```python
from build123d import *
from OCP.BRepFilletAPI import BRepFilletAPI_MakeChamfer

# Parameters (mm, degrees)
SKETCH1_W           = 22
SKETCH1_H           = 72
BOSS_EXTRUDE1_DEPTH = 5
SKETCH2_W           = 7
SKETCH2_H           = 15
BOSS_EXTRUDE2_DEPTH = 40
CHAMFER1_SIZE       = 1
FILLET1_R           = 10
CUT_EXTRUDE2_DEPTH  = 59.668560575
SKETCH6_W           = 7.5
SKETCH6_H           = 7.5
CUT_EXTRUDE3_DEPTH  = 55.927224579
CHAMFER2_SIZE2      = 15
CHAMFER2_SIZE       = 7.5
CHAMFER7_SIZE       = 7.5
CHAMFER3_SIZE       = 5
CUT_EXTRUDE6_DEPTH  = 2
CUT_EXTRUDE7_DEPTH  = 4
CHAMFER4_SIZE       = 2
CHAMFER4_SIZE_2     = 0.727940469
CUT_EXTRUDE8_DEPTH  = 60.42432162
CHAMFER8_SIZE2      = 7.5
CHAMFER8_SIZE       = 15
SKETCH12_R          = 1.7145
CUT_EXTRUDE9_DEPTH  = 60.42432162
SKETCH13_R          = 1.7145
CUT_EXTRUDE10_DEPTH = 55.927224579


with BuildPart() as part:
    # Sketch1 → Boss-Extrude1 (new body)
    with BuildSketch(Plane(origin=(0, 0, 0), x_dir=(1, 0, 0), z_dir=(0, 1, 0))):
        Rectangle(SKETCH1_W, SKETCH1_H)
    extrude(amount=BOSS_EXTRUDE1_DEPTH)

    # Sketch2 → Boss-Extrude2 (add)
    with BuildSketch(Plane(origin=(0, 5, 0), x_dir=(1, 0, 0), z_dir=(0, 1, 0))):
        with Locations((0, -28.5)):
            Rectangle(SKETCH2_W, SKETCH2_H)
    extrude(amount=BOSS_EXTRUDE2_DEPTH)

    # Chamfer1
    chamfer1_edges = [part.edges().sort_by_distance(p)[0] for p in [
        (0, 45, 36),
        (0, 45, 21),
    ]]
    chamfer(chamfer1_edges, length=CHAMFER1_SIZE)

    # Fillet1
    fillet1_edges = [part.edges().sort_by_distance(p)[0] for p in [
        (0, 5, 21),
    ]]
    fillet(fillet1_edges, radius=FILLET1_R)

    # Sketch5 → Cut-Extrude2 (cut, through all)
    with BuildSketch(Plane.XZ):
        with BuildLine():
            Line((3.4, 2), (3.4, -18))
            ThreePointArc((3.4, -18), (0, -21.4), (-3.4, -18))
            Line((-3.4, -18), (-3.4, 2))
            ThreePointArc((-3.4, 2), (0, 5.4), (3.4, 2))
        make_face()
    extrude(amount=-CUT_EXTRUDE2_DEPTH, mode=Mode.SUBTRACT)

    # Sketch6 → Cut-Extrude3 (cut, through all)
    with BuildSketch(Plane(origin=(0, 5, 0), x_dir=(1, 0, 0), z_dir=(0, 1, 0))):
        with Locations((7.25, -32.25)):
            Rectangle(SKETCH6_W, SKETCH6_H)
    cut_extrude3 = extrude(amount=-CUT_EXTRUDE3_DEPTH, mode=Mode.SUBTRACT)

    # Mirror1: Cut-Extrude3 across plane
    add(cut_extrude3.mirror(Plane(origin=(0, 0, 0), x_dir=(0, 0, 1), z_dir=(1, 0, 0))), mode=Mode.SUBTRACT)

    # Chamfer2
    chamfer2_edges = [part.edges().sort_by_distance(p)[0] for p in [
        (11, 2.5, 28.5),
    ]]
    chamfer2_side = [part.faces().sort_by_distance(p)[0] for p in [
        (10.85, 2.5, 28.5),
    ]]
    chamfer(chamfer2_edges, length=CHAMFER2_SIZE - 0.0001, length2=CHAMFER2_SIZE2 - 0.0001, reference=chamfer2_side[0])  # a hair under: the kernel refuses the full size

    # Chamfer7
    chamfer7_edges = [part.edges().sort_by_distance(p)[0] for p in [
        (0, 0, 36),
    ]]
    chamfer(chamfer7_edges, length=CHAMFER7_SIZE)

    # Chamfer3
    chamfer3_edges = [part.edges().sort_by_distance(p)[0] for p in [
        (-11, 2.5, -36),
        (11, 2.5, -36),
    ]]
    chamfer(chamfer3_edges, length=CHAMFER3_SIZE)

    # Sketch8 → Cut-Extrude6 (cut)
    # profile 1 of 2: a face of its own
    with BuildSketch(Plane.XZ):
        with BuildLine():
            Line((8.5, -18), (8.5, 2))
            ThreePointArc((8.5, 2), (0.500870333, 10.485230045), (-8.440971508, 3))
            Line((-8.440971508, 3), (-6, 3))
            Line((-6, 3), (-6, -19))
            Line((-6, -19), (-8.440971508, -19))
            ThreePointArc((-8.440971508, -19), (0.500870333, -26.485230045), (8.5, -18))
        make_face()
        with BuildLine():
            Line((-3.4, -18), (-3.4, 2))
            ThreePointArc((-3.4, 2), (0, 5.4), (3.4, 2))
            Line((3.4, 2), (3.4, -18))
            ThreePointArc((3.4, -18), (0, -21.4), (-3.4, -18))
        make_face(mode=Mode.SUBTRACT)
    # profile 2 of 2: a face of its own
    with BuildSketch(Plane.XZ):
        with BuildLine():
            Line((-6, 3), (-8.440971508, 3))
            ThreePointArc((-8.440971508, 3), (-8.485230045, 2.500870333), (-8.5, 2))
            Line((-8.5, 2), (-8.5, -18))
            ThreePointArc((-8.5, -18), (-8.485230045, -18.500870333), (-8.440971508, -19))
            Line((-8.440971508, -19), (-6, -19))
            Line((-6, -19), (-6, 3))
        make_face()
    extrude(amount=-CUT_EXTRUDE6_DEPTH, mode=Mode.SUBTRACT)

    # Sketch8<3> → Cut-Extrude7 (cut)
    with BuildSketch(Plane.XZ):
        with BuildLine():
            Line((-6, 3), (-8.440971508, 3))
            ThreePointArc((-8.440971508, 3), (-8.485230045, 2.500870333), (-8.5, 2))
            Line((-8.5, 2), (-8.5, -18))
            ThreePointArc((-8.5, -18), (-8.485230045, -18.500870333), (-8.440971508, -19))
            Line((-8.440971508, -19), (-6, -19))
            Line((-6, -19), (-6, 3))
        make_face()
    extrude(amount=-CUT_EXTRUDE7_DEPTH, mode=Mode.SUBTRACT)

    # Chamfer4
    chamfer4_edges_1 = [part.edges().sort_by_distance(p)[0] for p in [
        (8.5, 0, -8),
    ]]
    chamfer4_side_1 = [part.faces().sort_by_distance(p)[0] for p in [
        (8.5, 0.014558809, -8),
    ]]
    chamfer4_edges_2 = [part.edges().sort_by_distance(p)[0] for p in [
        (0, 0, -26.5),
    ]]
    chamfer4_side_2 = [part.faces().sort_by_distance(p)[0] for p in [
        (0, 0, -26.514558809),
    ]]
    chamfer4_edges_3 = [part.edges().sort_by_distance(p)[0] for p in [
        (0, 0, 10.5),
    ]]
    chamfer4_side_3 = [part.faces().sort_by_distance(p)[0] for p in [
        (0, 0, 10.514558809),
    ]]
    chamfer4_edges_4 = [part.edges().sort_by_distance(p)[0] for p in [
        (-8.5, 0, -8),
    ]]
    chamfer4_side_4 = [part.faces().sort_by_distance(p)[0] for p in [
        (-8.514558809, 0, -8),
    ]]
    chamfer4 = BRepFilletAPI_MakeChamfer(part.part.solid().wrapped)
    for e in chamfer4_edges_1:
        chamfer4.Add(CHAMFER4_SIZE - 0.0001, CHAMFER4_SIZE_2 - 0.0001, e.wrapped, chamfer4_side_1[0].wrapped)
    for e in chamfer4_edges_2:
        chamfer4.Add(CHAMFER4_SIZE - 0.0001, CHAMFER4_SIZE_2 - 0.0001, e.wrapped, chamfer4_side_2[0].wrapped)
    for e in chamfer4_edges_3:
        chamfer4.Add(CHAMFER4_SIZE - 0.0001, CHAMFER4_SIZE_2 - 0.0001, e.wrapped, chamfer4_side_3[0].wrapped)
    for e in chamfer4_edges_4:
        chamfer4.Add(CHAMFER4_SIZE - 0.0001, CHAMFER4_SIZE_2 - 0.0001, e.wrapped, chamfer4_side_4[0].wrapped)
    add(Compound.cast(chamfer4.Shape()), mode=Mode.REPLACE)  # a hair under: the kernel refuses the full size

    # Sketch9 → Cut-Extrude8 (cut, through all)
    with BuildSketch(Plane.ZY.offset(3.5)):
        with BuildLine():
            Line((26.7855, 20), (26.7855, 40))
            ThreePointArc((26.7855, 40), (28.5, 41.7145), (30.2145, 40))
            Line((30.2145, 40), (30.2145, 20))
            ThreePointArc((30.2145, 20), (28.5, 18.2855), (26.7855, 20))
        make_face()
    extrude(amount=-CUT_EXTRUDE8_DEPTH, mode=Mode.SUBTRACT)

    # Chamfer8
    chamfer8_edges = [part.edges().sort_by_distance(p)[0] for p in [
        (-11, 2.5, 28.5),
    ]]
    chamfer8_side = [part.faces().sort_by_distance(p)[0] for p in [
        (-11, 2.5, 28.35),
    ]]
    chamfer(chamfer8_edges, length=CHAMFER8_SIZE - 0.0001, length2=CHAMFER8_SIZE2 - 0.0001, reference=chamfer8_side[0])  # a hair under: the kernel refuses the full size

    # Sketch12 → Cut-Extrude9 (cut, through all)
    with BuildSketch(Plane(origin=(3.5, 0, 0), x_dir=(0, 0, -1), z_dir=(1, 0, 0))):
        with Locations((-28.5, 10)):
            Circle(SKETCH12_R)
    extrude(amount=-CUT_EXTRUDE9_DEPTH, mode=Mode.SUBTRACT)

    # Sketch13 → Cut-Extrude10 (cut, through all)
    with BuildSketch(Plane(origin=(0, 5, 0), x_dir=(1, 0, 0), z_dir=(0, 1, 0))):
        with Locations(Location((-7.25, -13.5, 0), (0, 0, 270))):
            Circle(SKETCH13_R)
        with Locations(Location((7.25, -13.5, 0), (0, 0, 270))):
            Circle(SKETCH13_R)
        with Locations(Location((-7.25, 28.5, 0), (0, 0, 270))):
            Circle(SKETCH13_R)
        with Locations(Location((7.25, 28.5, 0), (0, 0, 270))):
            Circle(SKETCH13_R)
    extrude(amount=-CUT_EXTRUDE10_DEPTH, mode=Mode.SUBTRACT)


solid = part.part
```
Build history of the part. All positions in model axes, mm. A direction names the side the tool comes from. Give positions to 0.01 mm unless a question says otherwise; leave off trailing zeros. Loops run counter-clockwise (first coordinate to the right, second up) from the corner with the lowest first, then second, coordinate; pieces in that order, holes last. Notation, with made-up numbers: (40.25, 24) - (62.25, 24) arc R17 cw to (62.25, 30) - close; hole circle Ø2 at (43, -1). An arc over 180 degrees is marked (long way). Use a Markdown table: item, result.
(1) Band-saw the part on B-B (y = 31). Give the cut face in (x, z).
Taken from the geometry:
| item | result |
|---|---|
| outline | (-3.5, 21) - (3.5, 21) - (3.5, 26.79) - (-3.5, 26.79) - close; (-3.5, 30.21) - (3.5, 30.21) - (3.5, 36) - (-3.5, 36) - close |
(2) Pull direction Z, two halves, no side cores. Call faces 4 (the face through (-7.907, 2.535, -26.916)), 5 (the face through (7.3, 2.5, 20.9)), 6 (the face through (0, 45, 28)): +Z half, -Z half, draft (parallel to the pull), parting line (faces both ways), or undercut.
Taken from the geometry:
| item | result |
|---|---|
| face 4 | undercut |
| face 5 | +Z half |
| face 6 | draft |
(3) Which spindle directions (+Z, -Z, +X, -X, +Y, -Y) get a long thin tool onto all of the face, cutting with end or side? Do faces 1 (the face through (-3.4, 3, -8)), 2 (the face through (0, 29, 21)), 3 (the face through (8.869, 0.986, -8.14)). Say none if no direction does.
Taken from the geometry:
| item | result |
|---|---|
| face 1 | +Y, -Y |
| face 2 | -Z, +X, -X, +Y |
| face 3 | -Y |
(4) Drop flat-ended pins along their axis: pin 1 Ø6 at (y, z) = (27.5, 26) entering from +X; pin 2 Ø1.6 at (x, y) = (-7.5, 3) entering from +Z; pin 3 Ø5 at (x, y) = (-5, 23.5) entering from -Z. Give the stop position or say it passes through.
Taken from the geometry:
| item | result |
|---|---|
| pin 1 | x = 3.5 |
| pin 2 | z = 22.1 |
| pin 3 | z = 21 |
(5) Wall check: line 1 along X through (y, z) = (1.65, -28.5); line 2 along Y through (x, z) = (-0.5, 28.5); line 3 along X through (y, z) = (3, -28). Give the ranges that are in metal, low to high.
Taken from the geometry:
| item | result |
|---|---|
| line 1 | -11 to -8.96, -5.54 to 5.54, 8.96 to 11 |
| line 2 | 0 to 8.29, 11.71 to 18.29, 41.71 to 45 |
| line 3 | -11 to -8.89, -5.61 to 5.61, 8.89 to 11 |
(6) Band-saw the part on A-A (x = 0). Give the number of separate pieces and of enclosed holes in the cut face, and give its area (3 significant figures).
Taken from the geometry:
| item | result |
|---|---|
| separate pieces | 2 |
| enclosed holes | 2 |
| area | 709 mm2 |
(7) Band-saw the part on C-C (z = -28.5). Give the cut face in (x, y).
Taken from the geometry:
| item | result |
|---|---|
| outline | (-11, 0) - (-8.96, 0) - (-8.96, 5) - (-11, 5) - close; (-5.54, 0) - (5.54, 0) - (5.54, 5) - (-5.54, 5) - close; (8.96, 0) - (11, 0) - (11, 5) - (8.96, 5) - close |
